from build123d import *

# Parameters (mm, degrees)
F0_W      = 6.35
F0_H      = 6.35
F1_DEPTH  = 19.05
F2_W      = 6.35
F2_H      = 6.35
F3_DEPTH  = 19.05
F4_W      = 6.35
F4_H      = 6.35
F5_DEPTH  = 19.05
F6_W      = 6.35
F6_H      = 6.35
F7_DEPTH  = 19.05
F8_W      = 6.35
F8_H      = 6.35
F9_DEPTH  = 19.05
F10_W     = 6.35
F10_H     = 6.35
F11_DEPTH = 19.05
F12_W     = 6.35
F12_H     = 6.35
F13_DEPTH = 19.05


with BuildPart() as f1:
    # F0 (on Top) → F1 (new body)
    with BuildSketch(Plane.XY):
        with Locations((3.175, 3.175)):
            Rectangle(F0_W, F0_H)
    extrude(amount=F1_DEPTH)

    # F2 (on face) → F3 (join)
    with BuildSketch(Plane.XZ):
        with Locations((3.175, 15.875)):
            Rectangle(F2_W, F2_H)
    extrude(amount=-F3_DEPTH)

    # F4 (on face) → F5 (join)
    with BuildSketch(Plane.XY.offset(19.05)):
        with Locations((3.175, 15.875)):
            Rectangle(F4_W, F4_H)
    extrude(amount=-F5_DEPTH)

    # F6 (on face) → F7 (join)
    with BuildSketch(Plane(origin=(0, 0, 0), x_dir=(0, -1, 0), z_dir=(-1, 0, 0))):
        with Locations((-15.875, 3.175)):
            Rectangle(F6_W, F6_H)
    extrude(amount=-F7_DEPTH)

    # F8 (on face) → F9 (join)
    with BuildSketch(Plane(origin=(0, 0, 0), x_dir=(1, 0, 0), z_dir=(0, 0, -1))):
        with Locations((15.875, -15.875)):
            Rectangle(F8_W, F8_H)
    extrude(amount=-F9_DEPTH)

    # F10 (on face) → F11 (join)
    with BuildSketch(Plane(origin=(0, 19.05, 0), x_dir=(-1, 0, 0), z_dir=(0, 1, 0))):
        with Locations((-15.875, 15.875)):
            Rectangle(F10_W, F10_H)
    extrude(amount=-F11_DEPTH)

    # F12 (on face) → F13 (join)
    with BuildSketch(Plane.XY.offset(19.05)):
        with Locations((15.875, 3.175)):
            Rectangle(F12_W, F12_H)
    extrude(amount=-F13_DEPTH)


solid = f1.part
Geometry check sheet. Reference: the model listing, model coordinates, mm. A direction names the side the tool comes from. Give positions to 0.01 mm unless a question says otherwise; leave off trailing zeros. Write each loop counter-clockwise with the first axis right and the second up, starting at its lowest first coordinate (ties: lowest second). Pieces come first, ordered by that corner, then holes. Notation, with made-up numbers: M 62,72 L 90,72 A25 cw 90,94 Z; hole C 4,81 d9. An arc over 180 degrees is marked long. One line per question, with ' | ' between items.
1. Set-up check for faces 4 (the face through (6.35, 7, 14)), 5 (the face through (3, 9, 12.7)), 6 (the face through (9, 16, 6.35)), 7 (the face through (3, 0, 9)): record each of +Z, -Z, +X, -X, +Y, -Y from which the full face is reachable in a straight line by a thin tool's end or side.
Ans:
face 4: +Z, -Y | face 5: -Z, +X, -X | face 6: +Z, +Y, -Y | face 7: +Z, -Z, +X, -X, -Y
2. Gauge pin test, flat end, axial feed: pin 1 (3 mm diameter, centred on x = 4.5, y = 10, fed in from -Z). Record the tip position at first contact, or that the pin passes through.
Ans:
pin 1: z = 12.7
3. Cross-section at B-B (z = 14.5). Enter the section's corners in (x, y).
Ans:
outline: M 0,0 L 6.35,0 L 6.35,19.05 L 0,19.05 Z; M 12.7,0 L 19.05,0 L 19.05,19.05 L 12.7,19.05 Z
4. Cross-section at A-A (y = 9.5). Enter the section's corners in (x, z), plus the area to 3 significant figures.
Ans:
outline: M 0,12.7 L 6.35,12.7 L 6.35,19.05 L 0,19.05 Z; M 12.7,12.7 L 19.05,12.7 L 19.05,19.05 L 12.7,19.05 Z | area: 80.6 mm2
5. Scan lines: line 1 along X through (y, z) = (1.25, 7.5); line 2 along Y through (x, z) = (6.75, 1.25). Record each from-to range of solid material in increasing order. Write a range as from..to.
Ans:
line 1: 0..6.35, 12.7..19.05 | line 2: 12.7..19.05
6. Cross-section at D-D (x = 17). Enter the section's corners in (y, z).
Ans:
outline: M 0,0 L 6.35,0 L 6.35,12.7 L 12.7,12.7 L 12.7,0 L 19.05,0 L 19.05,19.05 L 0,19.05 Z
7. Mould release check, pull along Y, two halves, no side actions. Record for faces 1 (the face through (16, 9, 19.05)), 2 (the face through (9, 19.05, 5)), 3 (the face through (16, 6.35, 6)): released by +Y, released by -Y, zero draft, split by the parting line, or undercut.
Ans:
face 1: zero draft | face 2: released by +Y | face 3: undercut
8. Cross-section at C-C (z = 1.75). Enter the section's corners in (x, y).
Ans:
outline: M 0,0 L 6.35,0 L 6.35,6.35 L 0,6.35 Z; M 0,12.7 L 19.05,12.7 L 19.05,19.05 L 0,19.05 Z; M 12.7,0 L 19.05,0 L 19.05,6.35 L 12.7,6.35 Z
